Read the model definition and answer for the solid it produces. Units are mm, in the model's axes. A direction names the side the tool comes from. Coordinates: 2 decimals unless noted, no trailing zeros. Order: outer loops, then holes, each group sorted by start corner. A loop starts at its lowest first (then second) coordinate and runs counter-clockwise, first axis right, second up. Notation, with made-up numbers: M 10,44 L 23,44 A16 cw 23,72 Z; hole C 14,84 d1. An arc over 180 degrees is marked long. Put each result on its own line as item: value.
from build123d import *

# Parameters (mm, degrees)
SKETCH_1_R      = 4
EXTRUDE_1_DEPTH = 30
SKETCH_2_R      = 3
EXTRUDE_2_DEPTH = 10
EXTRUDE_START   = 10
SKETCH_3_R      = 3
EXTRUDE_3_DEPTH = 10


with BuildPart() as part:
    # 草图1 → 凸台-拉伸1 (new, symmetric)
    with BuildSketch(Plane(origin=(0, 0, 526.914147293), x_dir=(-1, 0, 0), z_dir=(0, 0, -1))):
        with Locations(Location((340.287512766, -246.15455511, 0), (0, 0, 90))):
            Circle(SKETCH_1_R)
    extrude(amount=EXTRUDE_1_DEPTH, both=True)

    # 草图2 → 凸台-拉伸2 (add)
    with BuildSketch(Plane(origin=(0, 0, 496.914147293), x_dir=(-1, 0, 0), z_dir=(0, 0, -1))):
        with Locations(Location((340.287512766, -246.15455511, 0), (0, 0, 90))):
            Circle(SKETCH_2_R)
    extrude(amount=EXTRUDE_2_DEPTH)

    # 草图3 → 凸台-拉伸3 (add)
    with BuildSketch(Plane.XY.offset(556.914147293).offset(EXTRUDE_START)):
        with Locations(Location((-340.287512766, -246.15455511, 0), (0, 0, 90))):
            Circle(SKETCH_3_R)
    extrude(amount=-EXTRUDE_3_DEPTH)


solid = part.part
Q1. A tool of negligible diameter and unlimited length cuts with its end or side. For faces 1 (the face through (-340, -246, 566.914)), 2 (the face through (-342.95, -244.77, 491.98)), 3 (the face through (-337, -246, 556.914)), from which of +Z, -Z, +X, -X, +Y, -Y can it reach the whole face along a straight path? Write none if from no direction.
Answers below:
face 1: +Z, +X, -X, +Y, -Y
face 2: -Z
face 3: +Z
Q2. Find section B-B on y = -244. Write down the section's boundary in (x, z), plus the area to 3 significant figures.
Answers below:
outline: M -343.66,496.91 L -342.38,496.91 L -342.38,486.91 L -338.2,486.91 L -338.2,496.91 L -336.92,496.91 L -336.92,556.91 L -338.2,556.91 L -338.2,566.91 L -342.38,566.91 L -342.38,556.91 L -343.66,556.91 Z
area: 488 mm^2
Q3. Consider line 1 along Z through (x, y) = (-338.75, -242.5); line 2 along X through (y, z) = (-246, 515); line 3 along X through (y, z) = (-248.75, 509). Determine where each line is inside the solid, lowest interval first.
Answers below:
line 1: z = 496.91 to 556.91
line 2: x = -344.28 to -336.29
line 3: x = -343.33 to -337.24
Q4. Find section C-C on z = 560.5. Write down the section's boundary in (x, y), plus the area to 3 significant figures.
Answers below:
outline: C -340.29,-246.15 d6
area: 28.3 mm^2
Q5. Given pin 1 (4 mm diameter, centred on x = -338, z = 556, fed in from -Y), flat-ended and moving along its own axis, determine where the tip first touches the part or whether it passes through.
Answers below:
pin 1: stops at y = -250.14
Q6. Find section A-A on x = -338.75. Write down the section's boundary in (y, z), plus the area to 3 significant figures.
Answers below:
outline: M -249.85,496.91 L -248.73,496.91 L -248.73,486.91 L -243.58,486.91 L -243.58,496.91 L -242.46,496.91 L -242.46,556.91 L -243.58,556.91 L -243.58,566.91 L -248.73,566.91 L -248.73,556.91 L -249.85,556.91 Z
area: 546 mm^2
Q7. Find section D-D on z = 526. Write down the section's boundary in (x, y), plus the area to 3 significant figures.
Answers below:
outline: C -340.29,-246.15 d8
area: 50.3 mm^2
